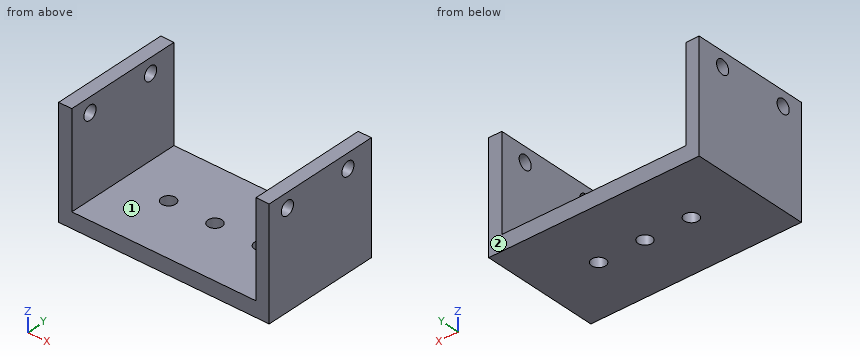
```python
from build123d import *

# Parameters (mm, degrees)
F0_W     = 42
F0_H     = 27
F2_DEPTH = 3.5
F0_W_2   = 3
F3_DEPTH = 25
F4_DEPTH = 25
F5_D     = 3.2
F5_DEPTH = 24.001
F6_D     = 3.2
F6_DEPTH = 24.001
F7_D     = 3.2


with BuildPart() as f2:
    # F0 (on Top) → F2 (new body)
    with BuildSketch(Plane.XY):
        Rectangle(F0_W, F0_H)
        with BuildLine():
            ThreePointArc((-12.175, 0), (-10.575, 1.6), (-8.975, 0))
            ThreePointArc((-8.975, 0), (-10.575, -1.6), (-12.175, 0))
        make_face(mode=Mode.SUBTRACT)
        with BuildLine():
            ThreePointArc((1.6, 0), (0, -1.6), (-1.6, 0))
            ThreePointArc((-1.6, 0), (0, 1.6), (1.6, 0))
        make_face(mode=Mode.SUBTRACT)
        with BuildLine():
            ThreePointArc((12.175, 0), (10.575, -1.6), (8.975, 0))
            ThreePointArc((8.975, 0), (10.575, 1.6), (12.175, 0))
        make_face(mode=Mode.SUBTRACT)
    extrude(amount=F2_DEPTH)

    # F0 (on Top) → F3 (join)
    with BuildSketch(Plane.XY):
        with Locations((-22.5, 0)):
            Rectangle(F0_W_2, F0_H)
    extrude(amount=F3_DEPTH)

    # F0 (on Top) → F4 (join)
    with BuildSketch(Plane.XY):
        with Locations((22.5, 0)):
            Rectangle(F0_W_2, F0_H)
    extrude(amount=F4_DEPTH)

    # F5 (through all, one way)
    with BuildSketch(Plane(origin=(0, 0, 0), x_dir=(0, 1, 0), z_dir=(-1, 0, 0))):
        with Locations((-8.6837460197, -21.689)):
            Circle(F5_D / 2)
    extrude(amount=-F5_DEPTH, mode=Mode.SUBTRACT)

    # F6 (through all, one way)
    with BuildSketch(Plane(origin=(0, 0, 0), x_dir=(0, 1, 0), z_dir=(-1, 0, 0))):
        with Locations((7.3162539803, -21.689)):
            Circle(F6_D / 2)
    extrude(amount=-F6_DEPTH, mode=Mode.SUBTRACT)

    # F7 (through all)
    with Locations(Plane.YZ):
        with Locations((-8.6837460197, 21.689), (7.3162539803, 21.689)):
            Hole(F7_D / 2)


solid = f2.part
```
CAD build for the part. Positions are in the model's coordinates, mm. Face numbers are marked on the shaded views. A direction names the side the tool comes from. Give positions to 0.01 mm unless a question says otherwise; leave off trailing zeros. Order: outer loops, then holes, each group sorted by start corner. A loop starts at its lowest first (then second) coordinate and runs counter-clockwise, first axis right, second up. Notation, with made-up numbers: M 39.5,-18 L 64.5,-18 A12 ccw 64.5,-7 Z; hole C 57.5,33.5 d1. An arc over 180 degrees is marked long. Put each result on its own line as item: value. Start each with the question number.
(1) Which spindle directions (+Z, -Z, +X, -X, +Y, -Y) get a long thin tool onto all of the face, cutting with end or side? Do the marked faces 1 and 2. Say none if no direction does.
(2) Drill centre lines: line 1 along X through (y, z) = (-7.5, 13.75); line 2 along Y through (x, z) = (0, 1.1); line 3 along X through (y, z) = (1.25, 1.5). Where is each one in solid material? Low to high.
(3) Saw through at A-A, the plane x = 0. Write the cut outline in (y, z).
(4) Saw through at B-B, the plane z = 15.25. Write the cut outline in (x, y).
(5) Saw through at C-C, the plane y = 0. Write the cut outline in (x, z) (3 decimals), then the cut area to 3 significant figures.
(6) Flat gauge pins, fed straight in: pin 1 Ø2.5 at (y, z) = (7.32, 21.69) entering from +X; pin 2 Ø6 at (x, y) = (-12, -6.5) entering from +Z. Where does each tip first touch, or does it go through?
(7) Saw through at D-D, the plane y = 4.5. Write the cut outline in (x, z), then the cut area to 3 significant figures.
Check result:
1. face 1: +Z, +Y, -Y
1. face 2: +Z, -Z, +X, -X, +Y
2. line 1: x = -24 to -21, 21 to 24
2. line 2: y = -13.5 to -1.6, 1.6 to 13.5
2. line 3: x = -24 to -11.57, -9.58 to -1, 1 to 9.58, 11.57 to 24
3. outline: M -13.5,0 L -1.6,0 L -1.6,3.5 L -13.5,3.5 Z; M 1.6,0 L 13.5,0 L 13.5,3.5 L 1.6,3.5 Z
4. outline: M -24,-13.5 L -21,-13.5 L -21,13.5 L -24,13.5 Z; M 21,-13.5 L 24,-13.5 L 24,13.5 L 21,13.5 Z
5. outline: M -24,0 L -12.175,0 L -12.175,3.5 L -21,3.5 L -21,25 L -24,25 Z; M -8.975,0 L -1.6,0 L -1.6,3.5 L -8.975,3.5 Z; M 1.6,0 L 8.975,0 L 8.975,3.5 L 1.6,3.5 Z; M 12.175,0 L 24,0 L 24,25 L 21,25 L 21,3.5 L 12.175,3.5 Z
5. area: 263 mm2
6. pin 1: passes through
6. pin 2: stops at z = 3.5
7. outline: M -24,0 L 24,0 L 24,25 L 21,25 L 21,3.5 L -21,3.5 L -21,25 L -24,25 Z
7. area: 297 mm2
